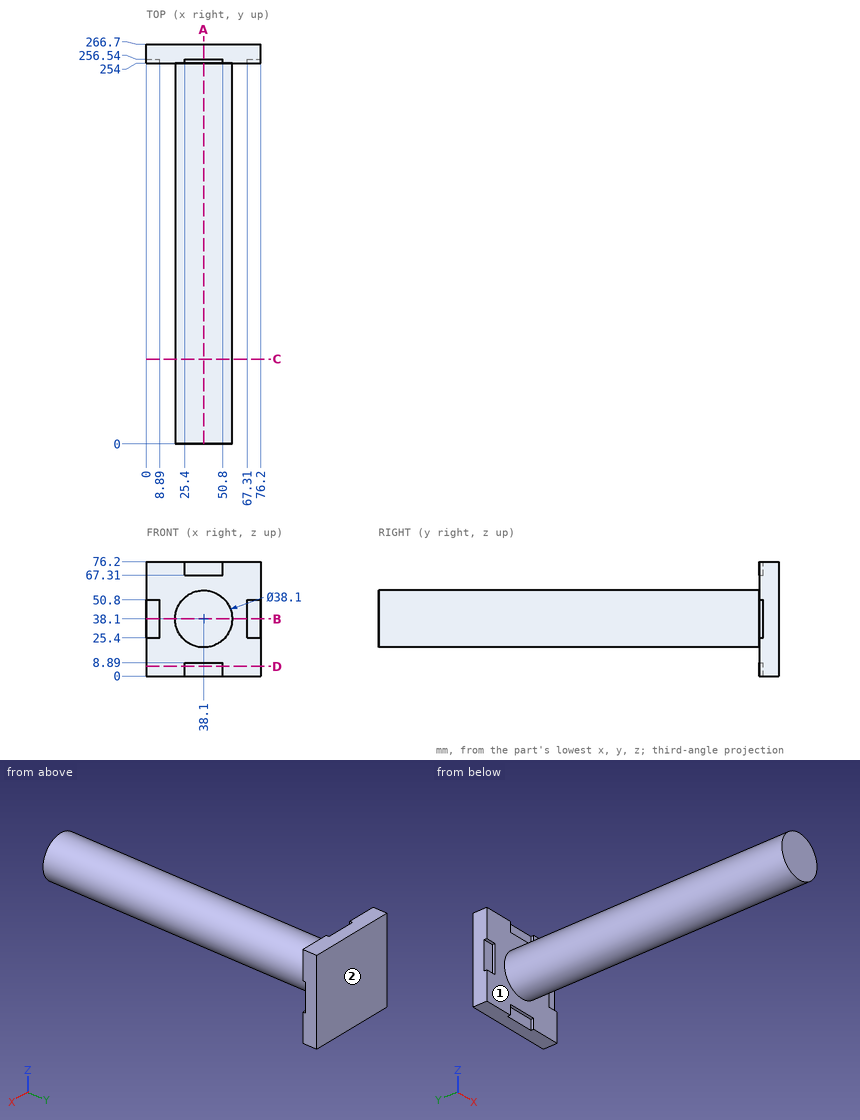
Check sheet for the drawn part. Datum: minimum x, y, z corner. Units: mm. A direction names the side the tool comes from. Round coordinates to 2 decimals unless told otherwise and drop trailing zeros. Order: outer loops, then holes, each group sorted by start corner. A loop starts at its lowest first (then second) coordinate and runs counter-clockwise, first axis right, second up.
(1) Cross-section at B-B, the plane z = 38.1. Enter the section's corners in (x, y), and give its area (3 significant figures).
(2) Go/stop test with flat-tipped pins: P1, Ø3, axis at x = 37, y = 255, coming from the -Z side; P2, Ø10, axis at x = 70.5, z = 39, coming from the -Y side; P3, Ø2, axis at x = 41.5, y = 113, coming from the -Z side. Record where each tip stops, or that it passes through.
(3) Cross-section at C-C, the plane y = 56.5. Enter the section's corners in (x, z), and give its area (3 significant figures).
(4) Cross-section at A-A, the plane x = 38.1. Enter the section's corners in (y, z), and give its area (3 significant figures).
(5) Access from +Z, -Z, +X, -X, +Y, -Y to the whole of each face (thin tool, end or side, straight path). Record for the marked faces 1 and 2.
(6) Cross-section at D-D, the plane z = 6.5. Enter the section's corners in (x, y), and give its area (3 significant figures).
(7) Scan lines: probe 1 along Y at (x, z) = (16, 73.5); probe 2 along Y at (x, z) = (4, 39.5); probe 3 along Z at (x, y) = (37, 148). Record each from-to range of solid material in increasing order.
Check sheet entries:
1. outline: (0, 256.54) - (8.89, 256.54) - (8.89, 254) - (19.05, 254) - (19.05, 0) - (57.15, 0) - (57.15, 254) - (67.31, 254) - (67.31, 256.54) - (76.2, 256.54) - (76.2, 266.7) - (0, 266.7) - close
1. area: 10,600 mm2
2. P1: stops at z = 8.89
2. P2: stops at y = 254
2. P3: stops at z = 19.2
3. outline: circle Ø38.1 at (38.1, 38.1)
3. area: 1,140 mm2
4. outline: (0, 19.05) - (254, 19.05) - (254, 8.89) - (256.54, 8.89) - (256.54, 0) - (266.7, 0) - (266.7, 76.2) - (256.54, 76.2) - (256.54, 67.31) - (254, 67.31) - (254, 57.15) - (0, 57.15) - close
4. area: 10,600 mm2
5. face 1: -Y
5. face 2: +Z, -Z, +X, -X, +Y
6. outline: (0, 254) - (25.4, 254) - (25.4, 256.54) - (50.8, 256.54) - (50.8, 254) - (76.2, 254) - (76.2, 266.7) - (0, 266.7) - close
6. area: 903 mm2
7. probe 1: y = 254 to 266.7
7. probe 2: y = 256.54 to 266.7
7. probe 3: z = 19.08 to 57.12
